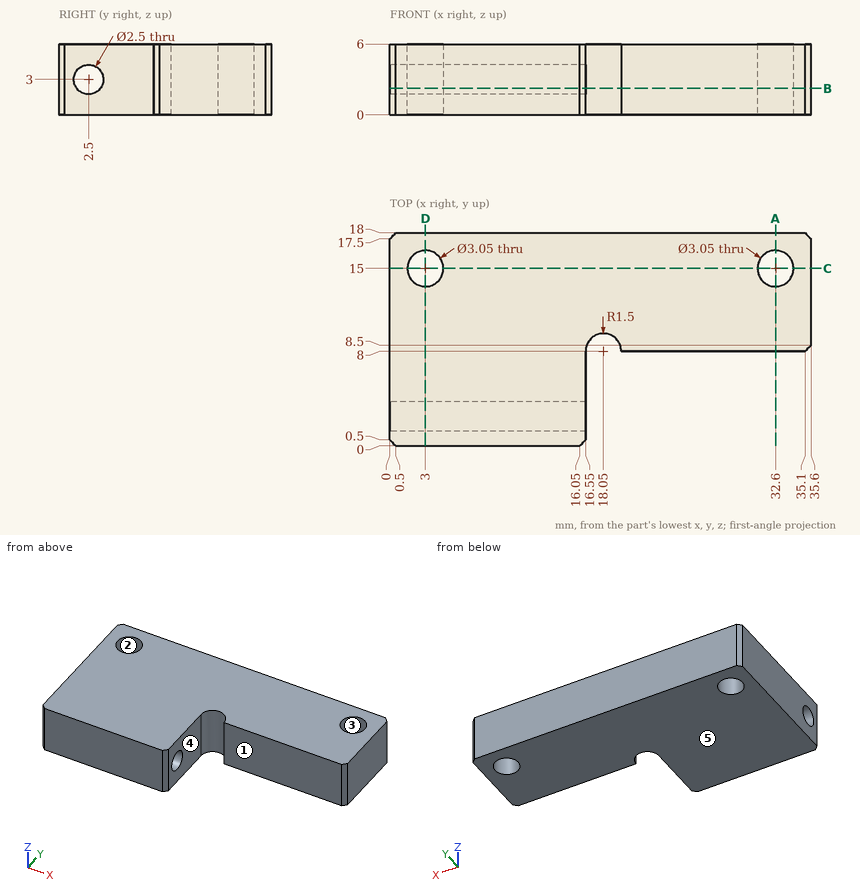
Job drawing, mm, ordinate dimensions from the low corner. One solid piece. A direction names the side the tool comes from. Round coordinates to 2 decimals unless told otherwise and drop trailing zeros. Loops run counter-clockwise (first coordinate to the right, second up) from the corner with the lowest first, then second, coordinate; pieces in that order, holes last.
(1) Which spindle directions (+Z, -Z, +X, -X, +Y, -Y) get a long thin tool onto all of the face, cutting with end or side? Do the marked faces 1 and 2. Say none if no direction does.
(2) Wall check: line 1 along Y through (x, z) = (32.6, 4.4) (3 decimals); line 2 along Y through (x, z) = (9.25, 3); line 3 along X through (y, z) = (14.25, 2.1). Give the ranges that are in metal, low to high.
(3) Two-plate mould, pull along X, no slides. Class the marked faces 3, 4 and 5: +X half, -X half, draft (parallel to the pull), parting line (faces both ways), or undercut.
(4) Cut at A-A (x = 32.6). Give the cut face in (y, z) (3 decimals).
(5) Cut at B-B (z = 2.25). Give the cut face in (x, y) (3 decimals).
(6) Drop flat-ended pins along their axis: pin 1 (1.5 mm diameter, centred on y = 2.5, z = 3, fed in from +X); pin 2 (3 mm diameter, centred on x = 29.5, z = 5, fed in from -Y). Give the stop position or say it passes through.
(7) Cut at D-D (x = 3). Give the cut face in (y, z) (3 decimals).
(8) Cut at C-C (y = 15). Give the cut face in (x, z) (3 decimals).
Findings below:
1. face 1: +Z, -Z, +X, -Y
1. face 2: +Z, -Z
2. line 1: y = 8 to 13.475, 16.525 to 18
2. line 2: y = 0 to 1.25, 3.75 to 18
2. line 3: x = 0 to 1.67, 4.33 to 31.27, 33.93 to 35.6
3. face 3: undercut
3. face 4: +X half
3. face 5: draft
4. outline: (8, 0) - (13.475, 0) - (13.475, 6) - (8, 6) - close; (16.525, 0) - (18, 0) - (18, 6) - (16.525, 6) - close
5. outline: (0, 0.5) - (0.5, 0) - (16.05, 0) - (16.55, 0.5) - (16.55, 1.5) - (0, 1.5) - close; (0, 3.5) - (16.55, 3.5) - (16.55, 8) arc R1.5 cw to (19.55, 8) - (35.1, 8) - (35.6, 8.5) - (35.6, 17.5) - (35.1, 18) - (0.5, 18) - (0, 17.5) - close; hole circle Ø3.05 at (3, 15); hole circle Ø3.05 at (32.6, 15)
6. pin 1: passes through
6. pin 2: stops at y = 8
7. outline: (0, 0) - (13.475, 0) - (13.475, 6) - (0, 6) - close; (16.525, 0) - (18, 0) - (18, 6) - (16.525, 6) - close; hole circle Ø2.5 at (2.5, 3)
8. outline: (0, 0) - (1.475, 0) - (1.475, 6) - (0, 6) - close; (4.525, 0) - (31.075, 0) - (31.075, 6) - (4.525, 6) - close; (34.125, 0) - (35.6, 0) - (35.6, 6) - (34.125, 6) - close
